The model under review builds one solid part; all positions refer to its coordinate system, in mm. A direction names the side the tool comes from. Coordinates: 2 decimals unless noted, no trailing zeros. Write each loop counter-clockwise with the first axis right and the second up, starting at its lowest first coordinate (ties: lowest second). Pieces come first, ordered by that corner, then holes. Notation, with made-up numbers: (40, 63.5) - (89, 63.5) arc R15 ccw to (89, 73.5) - close; hole circle Ø4 at (-11.5, 68.5). An arc over 180 degrees is marked (long way). Put each result on its own line as item: value.
from build123d import *

# Parameters (mm, degrees)
SKETCH2_W           = 1000
SKETCH2_H           = 150
SKETCH2_R           = 50
BOSS_EXTRUDE2_DEPTH = 100
SKETCH2_5_R         = 50
CUT_EXTRUDE1_DEPTH  = 30


with BuildPart() as part:
    # Sketch2 → Boss-Extrude2 (new body)
    with BuildSketch(Plane.XY):
        Rectangle(SKETCH2_W, SKETCH2_H)
        with Locations((-300, 0)):
            Circle(SKETCH2_R, mode=Mode.SUBTRACT)
        with Locations((300, 0)):
            Circle(SKETCH2_R, mode=Mode.SUBTRACT)
        Circle(SKETCH2_R, mode=Mode.SUBTRACT)
        with Locations((300, 0)):
            Circle(SKETCH2_R)
        Circle(SKETCH2_R)
        with Locations((-300, 0)):
            Circle(SKETCH2_R)
    extrude(amount=-BOSS_EXTRUDE2_DEPTH)

    # Sketch2_5 → Cut-Extrude1 (cut)
    with BuildSketch(Plane.XY):
        with Locations((-300, 0)):
            Circle(SKETCH2_5_R)
        with Locations((300, 0)):
            Circle(SKETCH2_5_R)
        Circle(SKETCH2_5_R)
    extrude(amount=-CUT_EXTRUDE1_DEPTH, mode=Mode.SUBTRACT)


solid = part.part
1. Machinability: for faces 5 (the flat face through (500, -1, -49)), 6 (the cylindrical face through (47.69, 15.02, -14.79)), which of the approach directions +Z, -Z, +X, -X, +Y, -Y give a long, thin tool a straight path to every point of the face, cutting with its end or side? Answer none if there is none.
Determined:
face 5: +Z, -Z, +X, +Y, -Y
face 6: +Z
2. The part is to be moulded in two halves that separate along Y. For faces 1 (the flat face through (-500, -1, -49)), 2 (the flat face through (-7, 75, -49)), 3 (the flat face through (-1, 1, -30)), 4 (the flat face through (-7, -75, -49)), say which applies: +Y half, -Y half, draft (parallel to the pull), parting line (faces both ways), or undercut.
Determined:
face 1: draft
face 2: +Y half
face 3: undercut
face 4: -Y half
3. To check wall thickness, follow probe 1 along X at (y, z) = (-4, -23); probe 2 along X at (y, z) = (16, -17); probe 3 along Z at (x, y) = (-303, -25). State the ranges of each line that lie inside material, in increasing order.
Determined:
probe 1: x = -500 to -349.84, -250.16 to -49.84, 49.84 to 250.16, 349.84 to 500
probe 2: x = -500 to -347.37, -252.63 to -47.37, 47.37 to 252.63, 347.37 to 500
probe 3: z = -100 to -30
4. Consider section B-B on y = 0. State the section outline as (x, z) points.
Determined:
outline: (-500, -100) - (500, -100) - (500, 0) - (350, 0) - (350, -30) - (250, -30) - (250, 0) - (50, 0) - (50, -30) - (-50, -30) - (-50, 0) - (-250, 0) - (-250, -30) - (-350, -30) - (-350, 0) - (-500, 0) - close
5. Consider section A-A on x = -300. State the section outline as (y, z) points.
Determined:
outline: (-75, -100) - (75, -100) - (75, 0) - (50, 0) - (50, -30) - (-50, -30) - (-50, 0) - (-75, 0) - close
6. For pin 1 Ø1.5 at (x, y) = (42.5, 11.5) entering from +Z, flat-tipped, find the tip position at first contact; note if it passes through.
Determined:
pin 1: stops at z = -30
